from build123d import *

# Parameters (mm, degrees)
BOSS_EXTRUDE1_DEPTH      = 20
BOSS_EXTRUDE2_DEPTH      = 1.5
BOSS_EXTRUDE2_DEPTH_BACK = 1.5


with BuildPart() as part:
    # Sketch1 → Boss-Extrude1 (new body)
    with BuildSketch(Plane(origin=(0, 0, 0), x_dir=(1, 0, 0), z_dir=(0, 1, 0))):
        Polygon((0, 0), (0, 10), (10, 10), (10, 0), (15, 0), (15, 20), (-5, 20), (-5, 0), align=None)
    extrude(amount=BOSS_EXTRUDE1_DEPTH)

    # Sketch3 → Boss-Extrude2 (add, two sides)
    with BuildSketch(Plane(origin=(5, 0, 0), x_dir=(0, 0, -1), z_dir=(1, 0, 0))) as boss_extrude2_sk:
        with BuildLine():
            Line((20, 18.912744364), (20, 19.412744364))
            ThreePointArc((20, 19.412744364), (22, 17.412744364), (20, 15.412744364))
            Line((20, 15.412744364), (20, 15.912744364))
            ThreePointArc((20, 15.912744364), (21.5, 17.412744364), (20, 18.912744364))
        make_face()
    extrude(amount=BOSS_EXTRUDE2_DEPTH)
    extrude(boss_extrude2_sk.sketch, amount=-BOSS_EXTRUDE2_DEPTH_BACK)


solid = part.part
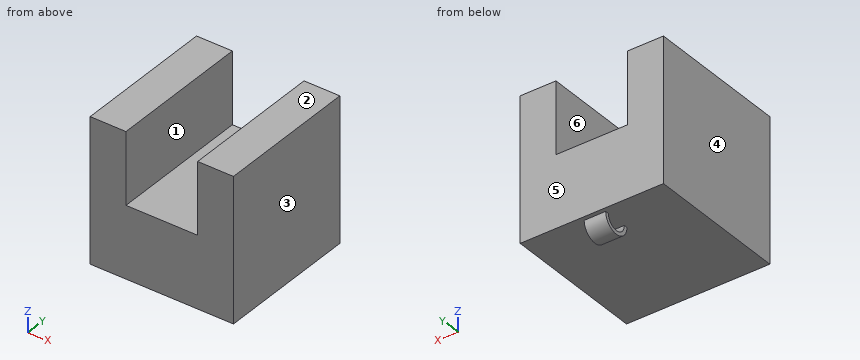
The model under review builds one solid part; all positions refer to its coordinate system, in mm. Face numbers are marked on the shaded views. A direction names the side the tool comes from. Coordinates: 2 decimals unless noted, no trailing zeros. Loops run counter-clockwise (first coordinate to the right, second up) from the corner with the lowest first, then second, coordinate; pieces in that order, holes last. Notation, with made-up numbers: M 62,44 L 100,44 A12 ccw 100,50 Z; hole C 48,-39 d2. An arc over 180 degrees is marked long. Put each result on its own line as item: value. Start each with the question number.
Q1. Add section C-C (y = 5). Write out the cut boundary in (x, z), and give its area (3 significant figures).
Q2. Add section B-B (y = 16.5). Write out the cut boundary in (x, z), and give its area (3 significant figures).
Q3. Add section D-D (x = -2.5). Write out the cut boundary in (y, z).
Q4. Add section A-A (z = -4.75). Write out the cut boundary in (x, y).
Q5. The part is to be moulded in two halves that separate along X. For the marked faces 3, 4, 5 and 6, say which applies: +X half, -X half, draft (parallel to the pull), parting line (faces both ways), or undercut.
Q6. Wall thickness on line 1 (X direction, y = 7.25, z = -8.5); line 2 (Z direction, x = 12, y = 3.25); line 3 (Z direction, x = 4.75, y = 14.5): over which ranges is each line inside the solid? List them lowest first.
Q7. For the marked faces 1 and 2, list the 3-axis set-ups (+Z, -Z, +X, -X, +Y, -Y) from which the entire face can be reached by the end or side of a thin tool; tool diameter is ignored.
Q8. Clearance check with flat-ended pins moving along their axes: pin 1 (1.5 mm diameter, centred on x = 3, y = 14.5, fed in from +Z); pin 2 (1.6 mm diameter, centred on y = 18, z = -21, fed in from +X); pin 3 (12 mm diameter, centred on x = 10.5, y = 8.5, fed in from -Z). State where each tip first meets the part, or that it passes through.
Answers:
1. outline: M -5,-20 L 15,-20 L 15,0 L 10,0 L 10,-10 L 0,-10 L 0,0 L -5,0 Z
1. area: 300 mm^2
2. outline: M -5,-20 L 15,-20 L 15,0 L 10,0 L 10,-10 L 0,-10 L 0,0 L -5,0 Z; M 3.5,-21.78 L 6.5,-21.78 L 6.5,-21.19 L 3.5,-21.19 Z
2. area: 302 mm^2
3. outline: M 0,-20 L 20,-20 L 20,0 L 0,0 Z
4. outline: M -5,0 L 0,0 L 0,20 L -5,20 Z; M 10,0 L 15,0 L 15,20 L 10,20 Z
5. face 3: +X half
5. face 4: -X half
5. face 5: draft
5. face 6: undercut
6. line 1: x = -5 to 0, 10 to 15
6. line 2: z = -20 to 0
6. line 3: z = -20 to -10
7. face 1: +Z, +Y, -Y
7. face 2: +Z, +X, -X, +Y, -Y
8. pin 1: stops at z = -10
8. pin 2: stops at x = 6.5
8. pin 3: stops at z = -20
